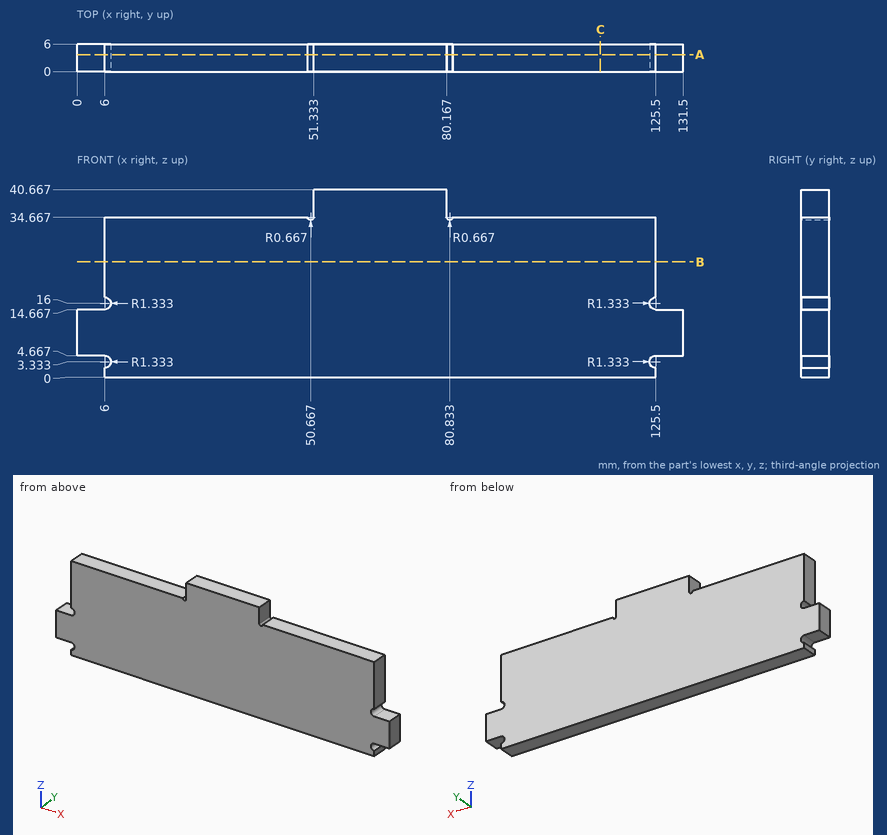
Drawing for the job (mm, zero at the part's lowest x, y, z). Give positions to 0.01 mm unless a question says otherwise; leave off trailing zeros. Loops run counter-clockwise (first coordinate to the right, second up) from the corner with the lowest first, then second, coordinate; pieces in that order, holes last.
1) Drop flat-ended pins along their axis: P1, Ø1, axis at y = 2, z = 0.5, coming from the +X side; P2, Ø3, axis at x = 2, y = 1.5, coming from the +Z side; P3, Ø3, axis at y = 2.5, z = 38.5, coming from the -X side. Give the stop position or say it passes through.
Values follow:
P1: stops at x = 125.5
P2: stops at z = 14.67
P3: stops at x = 51.33
2) Band-saw the part on C-C on x = 113.5. List the corners of the cut face in (y, z).
Values follow:
outline: (0, 0) - (6, 0) - (6, 34.67) - (0, 34.67) - close
3) Band-saw the part on A-A on y = 3.7. List the corners of the cut face in (x, z).
Values follow:
outline: (0, 4.67) - (6, 4.67) arc R1.33 cw to (6, 2) - (6, 0) - (125.5, 0) - (125.5, 2) arc R1.33 cw to (125.5, 4.67) - (131.5, 4.67) - (131.5, 14.67) - (125.5, 14.67) arc R1.33 cw to (125.5, 17.33) - (125.5, 34.67) - (81.5, 34.67) arc R0.67 cw to (80.17, 34.67) - (80.17, 40.67) - (51.33, 40.67) - (51.33, 34.67) arc R0.67 cw to (50, 34.67) - (6, 34.67) - (6, 17.33) arc R1.33 cw to (6, 14.67) - (0, 14.67) - close
4) Probe line 1 along Z through (x, y) = (6.5, 4.55) (1 decimal); line 2 along X through (y, z) = (0.95, 39); line 3 along Z through (x, y) = (83, 5.55). List the from-to ranges inside material, lowest first.
Values follow:
line 1: z = 0 to 2.1, 4.6 to 14.8, 17.2 to 34.7
line 2: x = 51.33 to 80.17
line 3: z = 0 to 34.67
5) Band-saw the part on B-B on z = 25. List the corners of the cut face in (x, y).
Values follow:
outline: (6, 0) - (125.5, 0) - (125.5, 6) - (6, 6) - close
